```python
from build123d import *

# Parameters (mm, degrees)
CROQUIS1_R              = 16.03
SALIENTE_EXTRUIR1_DEPTH = 9
CROQUIS2_R              = 10.5
SALIENTE_EXTRUIR2_DEPTH = 2
REDONDEO1_R             = 3
CROQUIS3_R              = 2
CORTAR_EXTRUIR1_DEPTH   = 44.150898021


with BuildPart() as part:
    # Croquis1 → Saliente-Extruir1 (new body)
    with BuildSketch(Plane.XY):
        with BuildLine():
            Line((-8.246211251, -16), (-25, -16))
            Line((-25, -16), (-25, -18))
            Line((-25, -18), (25, -18))
            Line((25, -18), (25, -16))
            Line((25, -16), (8.246211251, -16))
            ThreePointArc((8.246211251, -16), (0, 18), (-8.246211251, -16))
        make_face()
        Circle(CROQUIS1_R, mode=Mode.SUBTRACT)
    extrude(amount=SALIENTE_EXTRUIR1_DEPTH)

    # Croquis2 → Saliente-Extruir2 (add)
    with BuildSketch(Plane(origin=(0, 0, 0), x_dir=(-1, 0, 0), z_dir=(0, 0, -1))):
        with BuildLine():
            Line((-8.246211251, -16), (-25, -16))
            Line((-25, -16), (-25, -18))
            Line((-25, -18), (25, -18))
            Line((25, -18), (25, -16))
            Line((25, -16), (8.246211251, -16))
            ThreePointArc((8.246211251, -16), (0, 18), (-8.246211251, -16))
        make_face()
        Circle(CROQUIS2_R, mode=Mode.SUBTRACT)
    extrude(amount=-SALIENTE_EXTRUIR2_DEPTH)

    # Redondeo1
    redondeo1_edges = [part.edges().sort_by_distance(p)[0] for p in [
        (8.246211251, -16, 4.5),
        (-8.246211251, -16, 4.5),
    ]]
    fillet(redondeo1_edges, radius=REDONDEO1_R)

    # Croquis3 → Cortar-Extruir1 (cut, through all)
    with BuildSketch(Plane(origin=(0, -16, 0), x_dir=(1, 0, 0), z_dir=(0, 1, 0))):
        with Locations(Location((-21, -4.5, 0), (0, 0, 270))):
            Circle(CROQUIS3_R)
        with Locations(Location((21, -4.5, 0), (0, 0, 270))):
            Circle(CROQUIS3_R)
    extrude(amount=-CORTAR_EXTRUIR1_DEPTH, mode=Mode.SUBTRACT)


solid = part.part
```
Geometry: final body of the model. Coordinates: model frame, mm. A direction names the side the tool comes from. Round coordinates to 2 decimals unless told otherwise and drop trailing zeros. Order: outer loops, then holes, each group sorted by start corner. A loop starts at its lowest first (then second) coordinate and runs counter-clockwise, first axis right, second up. Notation, with made-up numbers: M -40,-23.75 L -36,-23.75 A21 ccw -36,-5.75 Z; hole C 32,-20 d4. An arc over 180 degrees is marked long. One line per item, written item: value.
(1) Cut plane C-C (z = 4.5). Return the cut outline in (x, y), and give its area (3 significant figures).
Result sheet:
outline: M -25,-18 L -23,-18 L -23,-16 L -25,-16 Z; M -19,-18 L 19,-18 L 19,-16 L 16.49,-16 A3 cw 14.14,-11.14 A18 ccw long -14.14,-11.14 A3 cw -16.49,-16 L -19,-16 Z; M 23,-18 L 25,-18 L 25,-16 L 23,-16 Z; hole C 0,0 d32.06
area: 295 mm2
(2) Pin query (flat end, axial travel): P1, Ø10, axis at x = 19, y = -12.5, coming from the +Z side; P2, Ø2, axis at x = 5, z = 4.5, coming from the +Y side; P3, Ø3.5, axis at x = -21, z = 4.5, coming from the -Y side; P4, Ø4, axis at x = 13.5, y = 3, coming from the +Z side. Return the tip coordinate at first contact, or that it passes through.
Result sheet:
P1: z = 9
P2: y = 17.55
P3: through
P4: z = 2
(3) Pull-direction query (Y, two-part tool) for faces 6 (the flat face through (0, -12, 0)), 7 (the flat face through (0, -18, 4)), 8 (the cylindrical face through (0.56, 17.99, 4.44)); classes: pulls with the +Y half, pulls with the -Y half, needs draft (parallel to the pull), parting line crosses it, or undercut.
Result sheet:
face 6: needs draft
face 7: pulls with the -Y half
face 8: undercut
(4) Reachability of faces 1 (the flat face through (-25, -17, 4)), 2 (the flat face through (-3.3, -10.5, 2)), 3 (the cylindrical face through (22.983, -16.986, 4.24)), 4 (the flat face through (21, -16, 2)), 5 (the flat face through (-18.8, -16, 4.4)) from +Z, -Z, +X, -X, +Y, -Y: full face, straight path, thin tool, end or side. Return the list, or none.
Result sheet:
face 1: +Z, -Z, -X, +Y, -Y
face 2: +Z
face 3: +Y, -Y
face 4: +Z, -Z, +X
face 5: +Z, -Z, -X
(5) Cut plane A-A (y = 0). Return the cut outline in (x, z).
Result sheet:
outline: M -18,0 L -10.5,0 L -10.5,2 L -16.03,2 L -16.03,9 L -18,9 Z; M 10.5,0 L 18,0 L 18,9 L 16.03,9 L 16.03,2 L 10.5,2 Z
(6) Cut plane D-D (z = 7). Return the cut outline in (x, y), and give its area (3 significant figures).
Result sheet:
outline: M -25,-18 L 25,-18 L 25,-16 L 16.49,-16 A3 cw 14.14,-11.14 A18 ccw long -14.14,-11.14 A3 cw -16.49,-16 L -25,-16 Z; hole C 0,0 d32.06
area: 311 mm2
(7) Line query: probe 1 along X at (y, z) = (0, 2.75); probe 2 along Y at (x, z) = (19, 3); probe 3 along X at (y, z) = (5, 7.75). Output: solid intervals per line, ascending. Write a range as [from, to].
Result sheet:
probe 1: [-18, -16.03], [16.03, 18]
probe 2: [-18, -16]
probe 3: [-17.29, -15.23], [15.23, 17.29]
